Part print with two shaded views. Sizes in mm from the minimum x, y, z corner. A direction names the side the tool comes from. Give positions to 0.01 mm unless a question says otherwise; leave off trailing zeros. Order: outer loops, then holes, each group sorted by start corner. A loop starts at its lowest first (then second) coordinate and runs counter-clockwise, first axis right, second up. Notation, with made-up numbers: M 13,-13.75 L 65,-13.75 A23 ccw 65,17.25 Z; hole C 19,68 d9. An arc over 180 degrees is marked long. Answer as CSV lines item,"result".
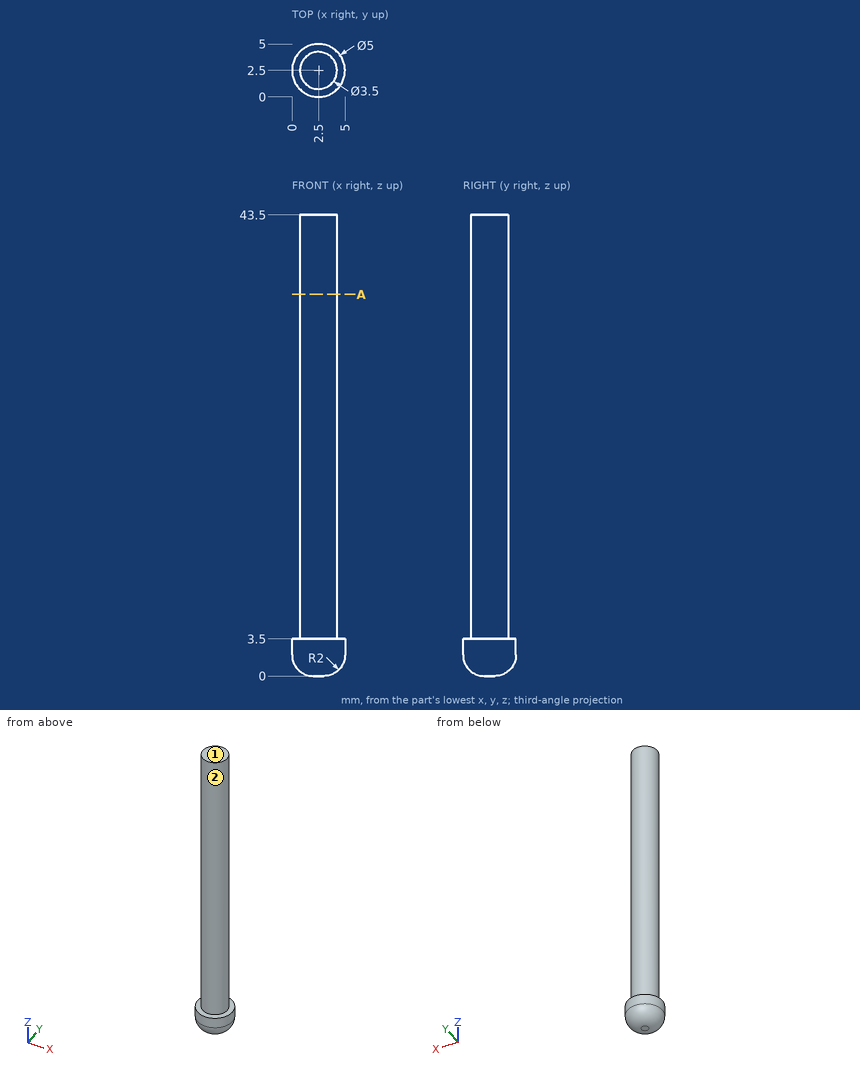
Item 1: Drop flat-ended pins along their axis: pin 1 (3 mm diameter, centred on y = 3.5, z = 33.5, fed in from +X); pin 2 (2 mm diameter, centred on x = 3, z = 32.5, fed in from -Y); pin 3 (1 mm diameter, centred on x = 4.5, y = 4, fed in from +Z). Give the stop position or say it passes through.
Geometry says:
pin 1,"stops at x = 4.25"
pin 2,"stops at y = 0.75"
pin 3,"stops at z = 3.5"
Item 2: 3-axis set-ups, long thin cutter, end or side, ignore diameter. For the marked faces 1 and 2: which of +Z, -Z, +X, -X, +Y, -Y reach the whole face in a straight line?
Geometry says:
face 1,"+Z, +X, -X, +Y, -Y"
face 2,"+Z"
Item 3: Probe line 1 along Y through (x, z) = (2.65, 30.5); line 2 along Z through (x, y) = (3.55, 0.8) (3 decimals). List the from-to ranges inside material, lowest first. Write a range as from..to.
Geometry says:
line 1,"y = 0.76..4.24"
line 2,"z = 0.675..3.5"
Item 4: Band-saw the part on A-A (z = 36). Give the cut face in (x, y).
Geometry says:
outline,"C 2.5,2.5 d3.5"
